Can you work these out from the drawing? Everything is in mm from the part's minimum corner. Coordinates: 2 decimals unless noted, no trailing zeros. Loops run counter-clockwise (first coordinate to the right, second up) from the corner with the lowest first, then second, coordinate; pieces in that order, holes last.
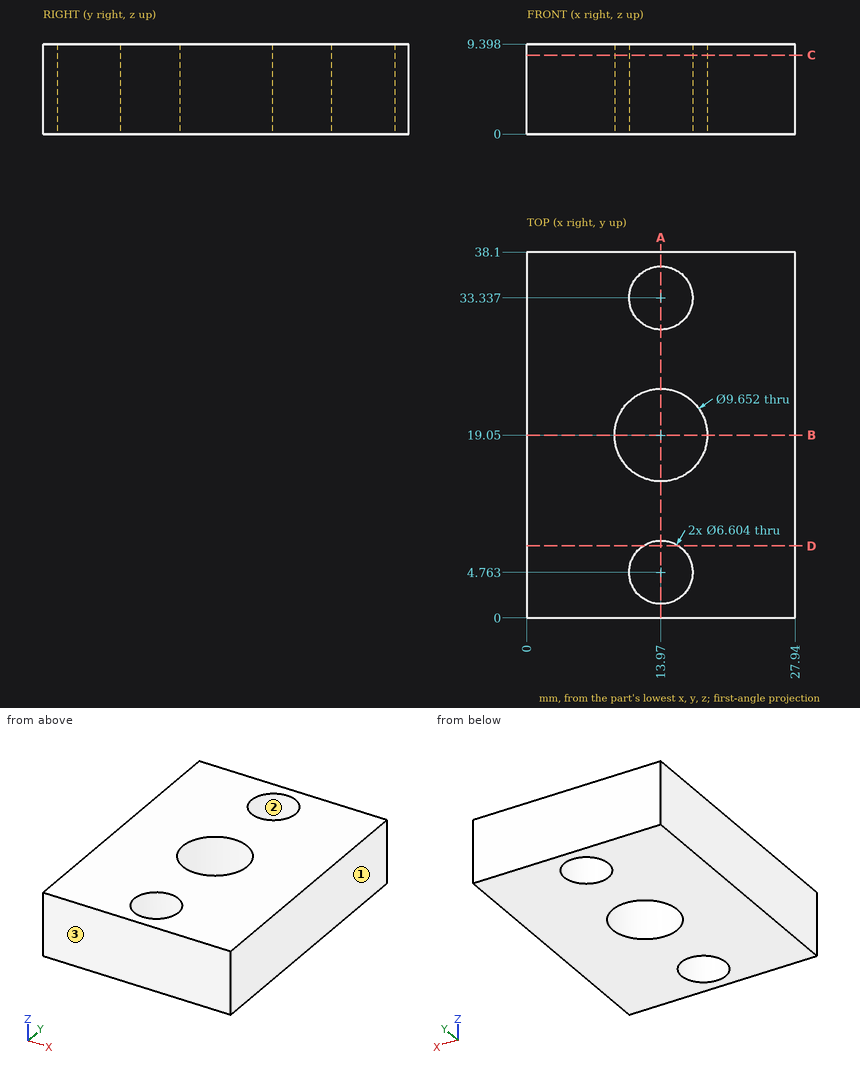
(1) Imagine slicing it at B-B, the plane y = 19.05. Write out the boundary of the cut face in (x, z) (1 decimal).
Answers:
outline: (0, 0) - (9.1, 0) - (9.1, 9.4) - (0, 9.4) - close; (18.8, 0) - (27.9, 0) - (27.9, 9.4) - (18.8, 9.4) - close
(2) We'd pull the mould along Y, two halves only. Please class the marked faces 1, 2 and 3: +Y half, -Y half, draft (parallel to the pull), parting line (faces both ways), or undercut.
Answers:
face 1: draft
face 2: undercut
face 3: -Y half
(3) I need wall thicknesses on probe 1 along Y at (x, z) = (13.97, 3.25) (1 decimal); probe 2 along X at (y, z) = (19.05, 4.75) (1 decimal); probe 3 along Y at (x, z) = (11.5, 5) (1 decimal). Which ranges of each line are inside material? Lowest first, please.
Answers:
probe 1: y = 0 to 1.5, 8.1 to 14.2, 23.9 to 30, 36.6 to 38.1
probe 2: x = 0 to 9.1, 18.8 to 27.9
probe 3: y = 0 to 2.6, 7 to 14.9, 23.2 to 31.1, 35.5 to 38.1
(4) Imagine slicing it at C-C, the plane z = 8.25. State how many separate pieces and enclosed holes the cut face has, and give its area (3 significant figures).
Answers:
separate pieces: 1
enclosed holes: 3
area: 923 mm2
(5) Imagine slicing it at A-A, the plane x = 13.97. Write out the boundary of the cut face in (y, z) (1 decimal).
Answers:
outline: (0, 0) - (1.5, 0) - (1.5, 9.4) - (0, 9.4) - close; (8.1, 0) - (14.2, 0) - (14.2, 9.4) - (8.1, 9.4) - close; (23.9, 0) - (30, 0) - (30, 9.4) - (23.9, 9.4) - close; (36.6, 0) - (38.1, 0) - (38.1, 9.4) - (36.6, 9.4) - close
(6) For pin 1 (5.5 mm diameter, centred on x = 13.97, y = 4.76, fed in from +Z) (3 decimals), with a flat end and sliding along its axis, tell me the tip position at first contact or that it passes through.
Answers:
pin 1: passes through
(7) Imagine slicing it at D-D, the plane y = 7.5. Write out the boundary of the cut face in (x, z), and give its area (3 significant figures).
Answers:
outline: (0, 0) - (12.12, 0) - (12.12, 9.4) - (0, 9.4) - close; (15.82, 0) - (27.94, 0) - (27.94, 9.4) - (15.82, 9.4) - close
area: 228 mm2
